For this review, use the dimensioned drawing (mm, ordinates from the lowest corner) and the shaded views. Give positions to 0.01 mm unless a question says otherwise; leave off trailing zeros. Order: outer loops, then holes, each group sorted by start corner. A loop starts at its lowest first (then second) coordinate and runs counter-clockwise, first axis right, second up. Notation, with made-up numbers: (69, 52) -> (118, 52) arc R26 cw to (118, 84) -> close; hole circle Ø8 at (18.5, -1). An arc over 180 degrees is marked (long way). One line per item, written item: value. Start each with the question number.
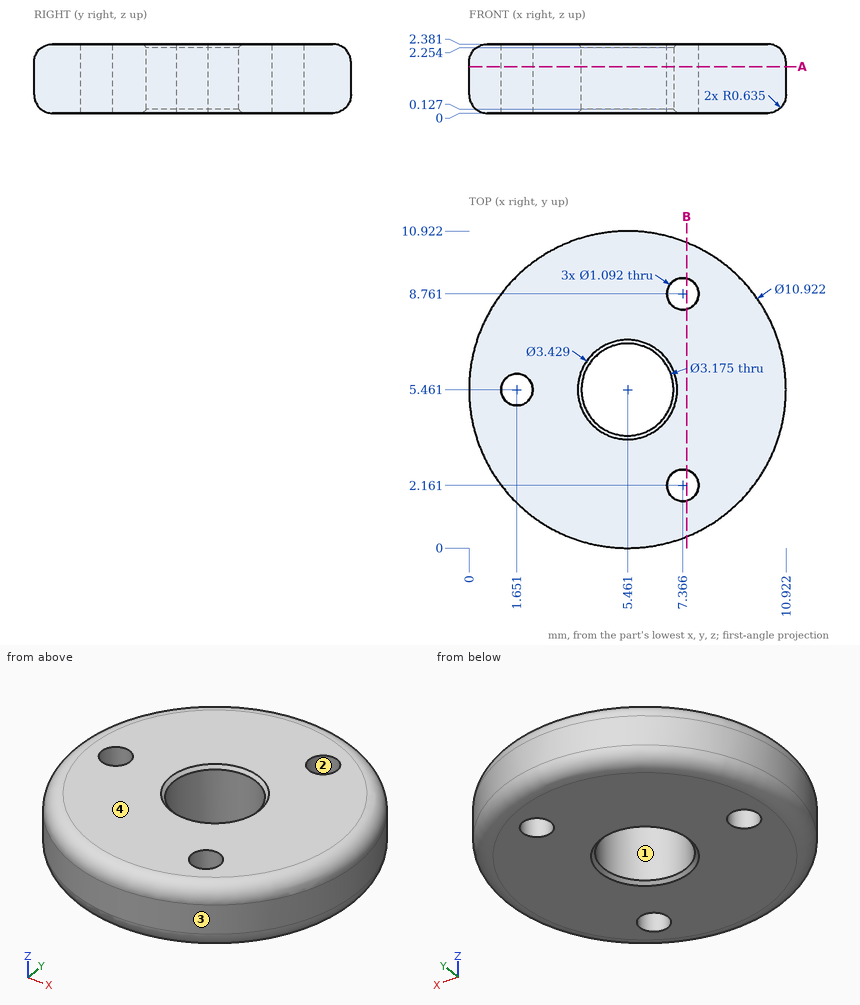
Q1. For line 1 along X through (y, z) = (6.5, 1.25); line 2 along Y through (x, z) = (6, 2.1) (1 decimal); line 3 along Y through (x, z) = (1.5, 2.15) (1 decimal), list the stretches that pass through material, from the lowest coordinate up.
Q2. Take a section at A-A (z = 1.6). State the section outline as (x, y) points (1 decimal).
Q3. For pin 1 Ø1.9 at (x, y) = (5.461, 5.461) entering from -Z; pin 2 Ø1 at (x, z) = (2, 1.5) entering from -Y, all flat-tipped, find the tip position at first contact; note any pin that passes through.
Q4. Take a section at B-B (x = 7.5). State how many separate pieces and enclosed holes the cut face has, and give its area (3 significant figures).
Q5. Mouldability with a two-part tool opening along X and no side actions: class the marked faces 1, 2, 3 and 4 as pulls with the +X half, pulls with the -X half, needs draft (parallel to the pull), parting line crosses it, or undercut.
Answers below:
1. line 1: x = 0.1 to 4.26, 6.66 to 10.82
1. line 2: y = 0.1 to 4, 7 to 10.8
1. line 3: y = 1.9 to 4.9, 6 to 9
2. outline: circle Ø10.9 at (5.5, 5.5); hole circle Ø1.1 at (1.7, 5.5); hole circle Ø3.2 at (5.5, 5.5); hole circle Ø1.1 at (7.4, 2.2); hole circle Ø1.1 at (7.4, 8.8)
3. pin 1: passes through
3. pin 2: stops at y = 0.87
4. separate pieces: 3
4. enclosed holes: 0
4. area: 18.7 mm²
5. face 1: undercut
5. face 2: undercut
5. face 3: parting line crosses it
5. face 4: needs draft
